Read the model definition and answer for the solid it produces. Units are mm, in the model's axes. A direction names the side the tool comes from. Give positions to 0.01 mm unless a question says otherwise; leave off trailing zeros. Write each loop counter-clockwise with the first axis right and the second up, starting at its lowest first coordinate (ties: lowest second). Pieces come first, ordered by that corner, then holes. Notation, with made-up numbers: (72.25, 13) - (79.25, 13) arc R24 cw to (79.25, 34) - close; hole circle Ø3 at (5.25, 63). An arc over 180 degrees is marked (long way). Answer as CSV lines item,"result".
```python
from build123d import *

# Parameters (mm, degrees)
F0_R         = 15
F0_R_2       = 12
F1_DEPTH     = 180
F2_DEPTH     = 160
F5_DEPTH     = 20
F6_DEPTH     = 18
F7_DEPTH     = 0.5
F8_DEPTH     = 160
F9_T1_DEPTH  = 33.1189779758
F10_T1_DEPTH = 33.1189779758
F11_R        = 1.6
F12_DEPTH    = 20


# Not quite as in the source:
# - a fillet or chamfer that OpenCascade refuses, or shapes differently, is made with other operations: its cross-section is extruded or revolved along the edge and cut away or added


with BuildPart() as f1:
    # F0 (on Front) → F1 (new body)
    with BuildSketch(Plane.XZ):
        Circle(F0_R)
        Circle(F0_R_2, mode=Mode.SUBTRACT)
        Circle(F0_R_2)
    extrude(amount=F1_DEPTH)

    # F0 (on Front) → F2 (cut)
    with BuildSketch(Plane.XZ):
        Circle(F0_R_2)
    extrude(amount=F2_DEPTH, mode=Mode.SUBTRACT)

    # F4 (on offset) → F5 (cut)
    with BuildSketch(Plane.XY.offset(-15)):
        with BuildLine():
            ThreePointArc((10.5, -117.0782160674), (5.5711218584, -114.3097131563), (0, -113.35))
            Line((0, -113.35), (0, -130))
            Line((0, -130), (7, -130))
            Line((7, -130), (10.5, -130))
            Line((10.5, -130), (10.5, -117.0782160674))
        make_face()
        with BuildLine():
            Line((0, -130), (0, -113.35))
            ThreePointArc((0, -113.35), (-5.5711218584, -114.3097131563), (-10.5, -117.0782160674))
            Line((-10.5, -117.0782160674), (-10.5, -130))
            Line((-10.5, -130), (-7, -130))
            Line((-7, -130), (0, -130))
        make_face()
    extrude(amount=F5_DEPTH, mode=Mode.SUBTRACT)

    # F4 (on offset) → F6 (join)
    with BuildSketch(Plane.XY.offset(-15)):
        with BuildLine():
            ThreePointArc((14.2855073516, -121.4474109355), (12.5838312774, -119.0972622529), (10.5, -117.0782160674))
            Line((10.5, -117.0782160674), (10.5, -130))
            Line((10.5, -130), (11.29, -130))
            Line((11.29, -130), (14.2855073516, -121.4474109355))
        make_face()
        with BuildLine():
            Line((-10.5, -130), (-10.5, -117.0782160674))
            ThreePointArc((-10.5, -117.0782160674), (-12.5838312774, -119.0972622529), (-14.2855073516, -121.4474109355))
            Line((-14.2855073516, -121.4474109355), (-11.29, -130))
            Line((-11.29, -130), (-10.5, -130))
        make_face()
    extrude(amount=F6_DEPTH)

    # F4 (on offset) → F7 (join)
    with BuildSketch(Plane.XY.offset(-15)):
        with BuildLine():
            Line((-10.5, -130), (-10.5, -117.0782160674))
            ThreePointArc((-10.5, -117.0782160674), (-12.5838312774, -119.0972622529), (-14.2855073516, -121.4474109355))
            Line((-14.2855073516, -121.4474109355), (-11.29, -130))
            Line((-11.29, -130), (-10.5, -130))
        make_face()
        with BuildLine():
            ThreePointArc((14.2855073516, -121.4474109355), (12.5838312774, -119.0972622529), (10.5, -117.0782160674))
            Line((10.5, -117.0782160674), (10.5, -130))
            Line((10.5, -130), (11.29, -130))
            Line((11.29, -130), (14.2855073516, -121.4474109355))
        make_face()
    extrude(amount=-F7_DEPTH)

    # F0 (on Front) → F8 (cut)
    with BuildSketch(Plane.XZ):
        Circle(F0_R_2)
    extrude(amount=F8_DEPTH, mode=Mode.SUBTRACT)

    # F9: chamfer of 3.9 x 2 on 1 edges, made by hand

    # F9_s2 → F9_t1 (cut)
    with BuildSketch(Plane.XZ.offset(106.9796190458)):
        Polygon((10.5, -13.5), (14.4, -15.5), (10.5, -15.5), align=None)
    extrude(amount=F9_T1_DEPTH, mode=Mode.SUBTRACT)

    # F10: chamfer of 2 x 3.9 on 1 edges, made by hand

    # F10_s2 → F10_t1 (cut)
    with BuildSketch(Plane.XZ.offset(106.9796190458)):
        Polygon((-10.5, -13.5), (-14.4, -15.5), (-10.5, -15.5), align=None)
    extrude(amount=F10_T1_DEPTH, mode=Mode.SUBTRACT)

    # F11 (on face) → F12 (cut)
    with BuildSketch(Plane.XZ.offset(180)):
        Circle(F11_R)
    extrude(amount=-F12_DEPTH, mode=Mode.SUBTRACT)


solid = f1.part
```
(1) A cutting plane is placed at B-B (x = 8). Write down the section's boundary in (y, z).
Worked out:
outline,"(-180, -12.69) - (-130, -12.69) - (-130, -8.94) - (-160, -8.94) - (-160, 8.94) - (0, 8.94) - (0, 12.69) - (-180, 12.69) - close; (-115.4, -12.69) - (0, -12.69) - (0, -8.94) - (-115.4, -8.94) - close"
(2) The mould has two halves that part along Z. Classify faces 1 (the flat face through (0, -130, -13)), 2 (the flat face through (11.946, -123.449, -14.241)), 3 (the flat face through (2, -160, 0)): +Z half, -Z half, draft (parallel to the pull), parting line (faces both ways), or undercut.
Worked out:
face 1,"draft"
face 2,"-Z half"
face 3,"undercut"
(3) For faces 4 (the flat face through (13.1, -124.83, -11.29)), 5 (the cylindrical face through (13, -119.6, -11.3)), 6 (the flat face through (10.5, -123, -10)), 7 (the flat face through (-11.946, -123.449, -14.241)), 8 (the flat face through (-13.142, -124.714, -11.139)), determine the directions among +Z, -Z, +X, -X, +Y, -Y from which every point of the face is accessible in a straight line to the end or side of a thin tool.
Worked out:
face 4,"-Z, +X, -Y"
face 5,"-Z, +X, +Y"
face 6,"-Z"
face 7,"-Z, +Y, -Y"
face 8,"-Z, -X, -Y"
(4) Each of these flat-tipped pins is pushed along its axis until it touches: P1, Ø2.5, axis at y = -123, z = -9, coming from the -X side; P2, Ø6, axis at y = -35, z = -12.5, coming from the +X side; P3, Ø2, axis at y = -38, z = 3, coming from the -X side. Where does it stop, or does it pass through?
Worked out:
P1,"stops at x = -14.18"
P2,"stops at x = 11.61"
P3,"stops at x = -14.87"
(5) A cutting plane is placed at A-A (z = 0). Write down the section's boundary in (x, y), and give its area (3 significant figures).
Worked out:
outline,"(-15, -180) - (-1.6, -180) - (-1.6, -160) - (-12, -160) - (-12, 0) - (-15, 0) - close; (1.6, -180) - (15, -180) - (15, 0) - (12, 0) - (12, -160) - (1.6, -160) - close"
area,"1,500 mm^2"
(6) Find the intervals of material crossed by L1, parallel to Z at x = 0, y = -85; L2, parallel to Z at x = 0, y = -169; L3, parallel to Y at x = -2, z = -4, in increasing order.
Worked out:
L1,"z = -15 to -12, 12 to 15"
L2,"z = -15 to -1.6, 1.6 to 15"
L3,"y = -180 to -160"
(7) A cutting plane is placed at C-C (y = -81). Write down the section's boundary in (x, z), and give its area (3 significant figures).
Worked out:
outline,"circle Ø30 at (0, 0); hole circle Ø24 at (0, 0)"
area,"254 mm^2"
